Model file for the job. Use its own axes, mm. A direction names the side the tool comes from. Round coordinates to 2 decimals unless told otherwise and drop trailing zeros. Loops run counter-clockwise (first coordinate to the right, second up) from the corner with the lowest first, then second, coordinate; pieces in that order, holes last. Notation, with made-up numbers: (7.5, 35.25) - (30.5, 35.25) arc R21 ccw to (30.5, 66.25) - close; hole circle Ø11 at (-24, 78.25). An arc over 180 degrees is marked (long way). Answer as a JSON object with one key per item and string values.
Autodesk Inventor part; units mm, degrees
ref_plane "YZ Plane" through (0, 0, 0) normal (1, 0, 0) x (0, 1, 0)
ref_plane "XZ Plane" through (0, 0, 0) normal (0, 1, 0) x (-1, 0, 0)
ref_plane "XY Plane" through (0, 0, 0) normal (0, 0, 1) x (1, 0, 0)
sketch "Sketch1" plane through (0, 0, 0) normal (0, 1, 0) x (-1, 0, 0)
  circle A0 centre (0, 0) radius 4
  dimension "d0" = 8
extrude "Extrusion1" add sketch "Sketch1" along normal blind 52
sketch "Sketch2" plane through (0, 52, 0) normal (0, 1, 0) x (1, 0, 0)
  point P0 (0, 0)
  point P1 (0, 0)
sketch "Sketch3" plane through (0, 0, 0) normal (0, -1, 0) x (1, 0, 0)
  point P0 (0, 0)
  point P1 (0, 0)
hole "Hole1" at (0, 52, 0) direction (0, -1, 0) diameter 3.4 depth 10.8 tip angle 118
hole "Hole2" at (0, 0, 0) direction (0, 1, 0) diameter 3.4 depth 10.8 tip angle 118
ref_plane "Work Plane2" through (0, 47, 0) normal (0, 1, 0) x (1, 0, 0)
ref_plane "Work Plane3" through (0, 26, 0) normal (0, 1, 0) x (1, 0, 0)
sketch "Sketch5" plane through (0, 47, 0) normal (0, 1, 0) x (1, 0, 0)
  circle A0 centre (0, 0) radius 2.75 construction
  line L0 (1.5877, 2.75) -> (3.1754, 0)
  line L1 (3.1754, 0) -> (1.5877, -2.75)
  line L2 (1.5877, -2.75) -> (-1.5877, -2.75)
  line L3 (-1.5877, -2.75) -> (-3.1754, 0)
  line L4 (-3.1754, 0) -> (-1.5877, 2.75)
  line L5 (-1.5877, 2.75) -> (1.5877, 2.75)
  point P0 (0, 2.75)
  dimension "d24" = 5.5
extrude "Extrusion3" cut sketch "Sketch5" against normal blind 2.48
mirror "Mirror2" about plane through (0, 26, 0) normal (0, 1, 0) of "Extrusion3"
properties part number "rod  for print"
1) Drop flat-ended pins along their axis: P1, Ø0.7, axis at x = 1, y = 6, coming from the +Z side; P2, Ø2, axis at y = 28, z = -3, coming from the +X side; P3, Ø1.2, axis at x = 1, y = 7, coming from the -Z side. Give the stop position or say it passes through.
Values follow:
{"P1": "z = 3.95", "P2": "x = 3.46", "P3": "z = -3.98"}
2) Two-plate mould, pull along Y, no slides. Class faces 1 (the flat face through (0, 6, -2.75)), 2 (the cylindrical face through (0.867, 25.636, 3.905)), 3 (the flat face through (-2, 52, 0)): pulls with the +Y half, pulls with the -Y half, needs draft (parallel to the pull), parting line crosses it, or undercut.
Values follow:
{"face 1": "undercut", "face 2": "needs draft", "face 3": "pulls with the +Y half"}
3) Slice it at B-B on y = 39. List the corners of the cut face in (x, z).
Values follow:
{"outline": "circle Ø8 at (0, 0)"}
4) Tool access for faces 4 (the flat face through (-2.39, 6.22, 1.36)), 5 (the cylindrical face through (1.66, 9.16, 0.37)), 6 (the cylindrical face through (1.66, 42.84, -0.37)): list every direction of +Z, -Z, +X, -X, +Y, -Y with a clear straight run to the whole face (end or side of a thin tool).
Values follow:
{"face 4": "none", "face 5": "-Y", "face 6": "+Y"}
5) Slice it at A-A on y = 4. List the corners of the cut face in (x, z), then the cut area to 3 significant figures.
Values follow:
{"outline": "circle Ø8 at (0, 0); hole circle Ø3.4 at (0, 0)", "area": "41.2 mm²"}
6) Probe probe 1 along Y at (x, z) = (1.75, 0); probe 2 along Z at (x, y) = (0, 3.7); probe 3 along Z at (x, y) = (0, 5.5). List the from-to ranges inside material, lowest first.
Values follow:
{"probe 1": "0 to 5, 7.48 to 44.52, 47 to 52", "probe 2": "-4 to -1.7, 1.7 to 4", "probe 3": "-4 to -2.75, 2.75 to 4"}
7) Slice it at C-C on z = 3.5. List the corners of the cut face in (x, y).
Values follow:
{"outline": "(-1.94, 0) - (1.94, 0) - (1.94, 52) - (-1.94, 52) - close"}
